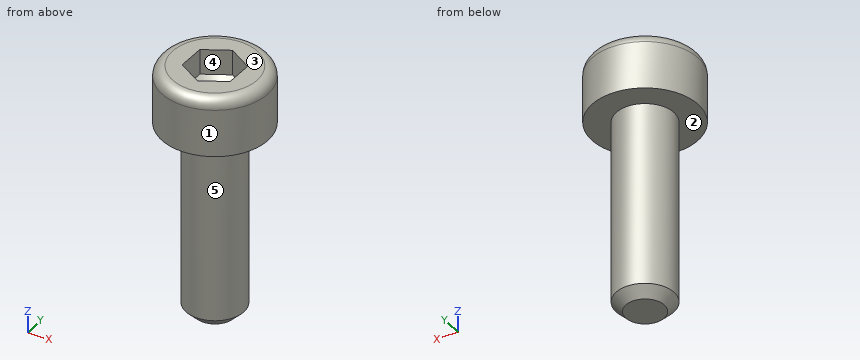
Solid Edge part; units mm, degrees
sketch "Sketch1" plane through (0, 0, 0) normal (0, -1, 0) x (1, 0, 0)
  line L0 (0, 0) -> (2.2, 0)
  arc A0 (2.2, 0) -> (2.75, -0.55) centre (2.2, -0.55) cw
  line L1 (2.75, -0.55) -> (2.75, -3)
  line L2 (2.75, -3) -> (1.5, -3)
  line L3 (1.5, -3) -> (1.5, -12.5)
  line L4 (1.5, -12.5) -> (1, -13)
  line L5 (1, -13) -> (0, -13)
revolve "RevolvedProtrusion1" add sketch "Sketch1" angle 360 about axis through (0, 0, -13) along (0, 0, 1)
sketch "Sketch2" plane through (0, 0, 0) normal (0, 0, 1) x (1, 0, 0)
  line L0 (-1.25, -0.7217) -> (-1.25, 0.7217)
  line L1 (-1.25, 0.7217) -> (0, 1.4434)
  line L2 (0, 1.4434) -> (1.25, 0.7217)
  line L3 (1.25, 0.7217) -> (1.25, -0.7217)
  line L4 (1.25, -0.7217) -> (0, -1.4434)
  line L5 (0, -1.4434) -> (-1.25, -0.7217)
extrude "Cutout1" cut sketch "Sketch2" against normal blind 1.3
sketch "Sketch3" plane through (0, 0, 0) normal (1, 0, 0) x (0, 1, 0)
  line L0 (0, -2.1333) -> (1.4434, -1.3)
  line L1 (0, -1.3) -> (1.4434, -1.3)
  line L2 (0, -1.3) -> (0, -2.1333)
revolve "RevolvedCutout1" cut sketch "Sketch3" angle 360 about axis through (0, 0, -60.325) along (0, 0, 1)
cosmetic_thread "Thread1"
properties part number "26"
Model file for the job. Use its own axes, mm. Face numbers are marked on the shaded views. A direction names the side the tool comes from. Coordinates: 2 decimals unless noted, no trailing zeros. Write each loop counter-clockwise with the first axis right and the second up, starting at its lowest first coordinate (ties: lowest second). Pieces come first, ordered by that corner, then holes. Notation, with made-up numbers: (-11.75, -2.75) -> (38.25, -2.75) arc R22 ccw to (38.25, 20.25) -> close; hole circle Ø4 at (33.25, 29). An arc over 180 degrees is marked (long way). One line per item, written item: value. Start each with the question number.
1) Flat gauge pin, fed straight in: pin 1 Ø2 at (y, z) = (-1.5, -4.5) entering from +X. Where does the tip first touch, or does it go through?
2) Which spindle directions (+Z, -Z, +X, -X, +Y, -Y) get a long thin tool onto all of the face, cutting with end or side? Do the marked faces 1 and 2. Say none if no direction does.
3) Slice it at A-A on z = -9.25. Write the cut outline in (x, y).
4) Probe probe 1 along Y at (x, z) = (0.4, -3.5); probe 2 along Y at (x, z) = (-2.45, -2.5); probe 3 along X at (y, z) = (0.7, -1.25). List the from-to ranges inside material, lowest first.
5) Pull direction Y, two halves, no side cores. Call the marked faces 3, 4 and 5: +Y half, -Y half, draft (parallel to the pull), parting line (faces both ways), or undercut.
Answers follow:
1. pin 1: x = 1.41
2. face 1: +Z, -Z
2. face 2: -Z
3. outline: circle Ø3 at (0, 0)
4. probe 1: -1.45 to 1.45
4. probe 2: -1.25 to 1.25
4. probe 3: -2.66 to -1.25, 1.25 to 2.66
5. face 3: draft
5. face 4: undercut
5. face 5: parting line
